from build123d import *

# Parameters (mm, degrees)
BOSS_EXTRU_1_DEPTH                    = 3.6
ESQUISSE2_W                           = 19.8
ESQUISSE2_H                           = 10.6
BOSS_EXTRU_2_DEPTH                    = 1.4
ESQUISSE3_W                           = 19.8
ESQUISSE3_H                           = 10.6
BOSS_EXTRU_3_DEPTH                    = 1.4
ESQUISSE4_W                           = 3.6
ESQUISSE4_H                           = 0.3
BOSS_EXTRU_4_DEPTH                    = 16.265607889
ESQUISSE5_W                           = 10.8
ESQUISSE5_H                           = 1.1
ENL_V_MAT_EXTRU_1_DEPTH               = 7.4
ESQUISSE6_W                           = 3.8
ESQUISSE6_H                           = 0.4
ENL_V_MAT_EXTRU_2_DEPTH               = 7.4
ESQUISSE7_W                           = 6.7
ESQUISSE7_H                           = 0.4
ENL_V_MAT_EXTRU_3_DEPTH               = 7.4
ESQUISSE8_W                           = 3.7
ESQUISSE8_H                           = 0.4
ENL_V_MAT_EXTRU_4_DEPTH               = 7.4
ENL_V_MAT_EXTRU_5_DEPTH               = 7.4
BOSS_EXTRU_5_DEPTH                    = 3.2
ESQUISSE11_W                          = 0.5
ESQUISSE11_H                          = 3.2
BOSS_EXTRU_6_DEPTH                    = 3.9
ESQUISSE12_W                          = 0.5
ESQUISSE12_H                          = 3.2
BOSS_EXTRU_7_DEPTH                    = 3.9
ESQUISSE13_W                          = 0.5
ESQUISSE13_H                          = 3.2
BOSS_EXTRU_8_DEPTH                    = 3.9
D_POUILLE1_ANGLE                      = 32.471192291
D_POUILLE2_ANGLE                      = 45
D_POUILLE3_ANGLE                      = 45
DIAM_TRE_DU_PER_AGE_2_35_2_35_1_D     = 2.35
DIAM_TRE_DU_PER_AGE_2_35_2_35_1_DEPTH = 6.4
CONG_1_R                              = 0.5
ESQUISSE16_R                          = 0.5
ENL_V_MAT_EXTRU_6_DEPTH               = 19.45


with BuildPart() as part:
    # Esquisse1 → Boss.-Extru.1 (new body)
    with BuildSketch(Plane(origin=(0, 0, -1.8), x_dir=(-1, 0, 0), z_dir=(0, 0, -1))):
        Polygon((7.1, 11.621125946), (6.88877818, 11.686563143), (6.8, 11.4), (6.8, 10.6), (-9.9, 10.6), (-9.9, 0), (9.9, 0), (9.9, 10.6), (7.1, 10.6), align=None)
    extrude(amount=-BOSS_EXTRU_1_DEPTH)

    # Esquisse2 → Boss.-Extru.2 (add)
    with BuildSketch(Plane(origin=(0, 0, -1.8), x_dir=(-1, 0, 0), z_dir=(0, 0, -1))):
        with Locations((0, 5.3)):
            Rectangle(ESQUISSE2_W, ESQUISSE2_H)
    extrude(amount=BOSS_EXTRU_2_DEPTH)

    # Esquisse3 → Boss.-Extru.3 (add)
    with BuildSketch(Plane.XY.offset(1.8)):
        with Locations((0, 5.3)):
            Rectangle(ESQUISSE3_W, ESQUISSE3_H)
    extrude(amount=BOSS_EXTRU_3_DEPTH)

    # Esquisse4 → Boss.-Extru.4 (add)
    with BuildSketch(Plane(origin=(-2.982033775, -0.923843615, 0), x_dir=(0, 0, -1), z_dir=(0.955210476, 0.295927265, 0))):
        with Locations((0, 13.051704831)):
            Rectangle(ESQUISSE4_W, ESQUISSE4_H)
    extrude(amount=BOSS_EXTRU_4_DEPTH)

    # Esquisse5 → Enlèv. mat.-Extru.1 (cut, through all)
    with BuildSketch(Plane.XY.offset(3.2)):
        with Locations((4.5, 10.05)):
            Rectangle(ESQUISSE5_W, ESQUISSE5_H)
    extrude(amount=-ENL_V_MAT_EXTRU_1_DEPTH, mode=Mode.SUBTRACT)

    # Esquisse6 → Enlèv. mat.-Extru.2 (cut, through all)
    with BuildSketch(Plane.XY.offset(3.2)):
        with Locations((8, 0.2)):
            Rectangle(ESQUISSE6_W, ESQUISSE6_H)
    extrude(amount=-ENL_V_MAT_EXTRU_2_DEPTH, mode=Mode.SUBTRACT)

    # Esquisse7 → Enlèv. mat.-Extru.3 (cut, through all)
    with BuildSketch(Plane.XY.offset(3.2)):
        with Locations((-0.05, 0.2)):
            Rectangle(ESQUISSE7_W, ESQUISSE7_H)
    extrude(amount=-ENL_V_MAT_EXTRU_3_DEPTH, mode=Mode.SUBTRACT)

    # Esquisse8 → Enlèv. mat.-Extru.4 (cut, through all)
    with BuildSketch(Plane.XY.offset(3.2)):
        with Locations((-8.05, 0.2)):
            Rectangle(ESQUISSE8_W, ESQUISSE8_H)
    extrude(amount=-ENL_V_MAT_EXTRU_4_DEPTH, mode=Mode.SUBTRACT)

    # Esquisse9 → Enlèv. mat.-Extru.5 (cut, through all)
    with BuildSketch(Plane.XY.offset(3.2)):
        with BuildLine():
            Line((-5.24, 1.73), (-4.36, 1.73))
            ThreePointArc((-4.36, 1.73), (-3.550086003, 2.914662921), (-4.387568187, 4.08))
            Line((-4.387568187, 4.08), (-5.212431813, 4.08))
            ThreePointArc((-5.212431813, 4.08), (-6.049913997, 2.914662921), (-5.24, 1.73))
        make_face()
    extrude(amount=-ENL_V_MAT_EXTRU_5_DEPTH, mode=Mode.SUBTRACT)

    # Esquisse10 → Boss.-Extru.5 (add)
    with BuildSketch(Plane(origin=(0, 0, -1.6), x_dir=(-1, 0, 0), z_dir=(0, 0, -1))):
        with BuildLine():
            Line((1.8, 10.6), (3.8, 10.6))
            Line((3.8, 10.6), (3.8, 11.263324958))
            ThreePointArc((3.8, 11.263324958), (2.8, 11.8), (1.8, 11.263324958))
            Line((1.8, 11.263324958), (1.8, 10.6))
        make_face()
    extrude(amount=-BOSS_EXTRU_5_DEPTH)

    # Esquisse11 → Boss.-Extru.6 (add)
    with BuildSketch(Plane.XZ.offset(-0.4)):
        with Locations((-8.3, 0)):
            Rectangle(ESQUISSE11_W, ESQUISSE11_H)
    extrude(amount=BOSS_EXTRU_6_DEPTH)

    # Esquisse12 → Boss.-Extru.7 (add)
    with BuildSketch(Plane.XZ.offset(-0.4)):
        with Locations((0.5, 0)):
            Rectangle(ESQUISSE12_W, ESQUISSE12_H)
    extrude(amount=BOSS_EXTRU_7_DEPTH)

    # Esquisse13 → Boss.-Extru.8 (add)
    with BuildSketch(Plane.XZ.offset(-0.4)):
        with Locations((7.8, 0)):
            Rectangle(ESQUISSE13_W, ESQUISSE13_H)
    extrude(amount=BOSS_EXTRU_8_DEPTH)

    # Dépouille1
    d_pouille1_faces = [part.faces().sort_by_distance(p)[0] for p in [
        (-0.9, 10.05, 0),
    ]]
    draft(d_pouille1_faces, Plane(origin=(-9.9, 10.6, 1.8), x_dir=(0, 0, 1), z_dir=(0, 1, 0)), D_POUILLE1_ANGLE)

    # Dépouille2
    d_pouille2_faces = [part.faces().sort_by_distance(p)[0] for p in [
        (6.1, 0.2, 0),
        (3.3, 0.2, 0),
    ]]
    draft(d_pouille2_faces, Plane(origin=(9.9, 0, 1.8), x_dir=(0, 0, -1), z_dir=(0, -1, 0)), D_POUILLE2_ANGLE)

    # Dépouille3
    d_pouille3_faces = [part.faces().sort_by_distance(p)[0] for p in [
        (-3.4, 0.2, 0),
        (-6.2, 0.2, 0),
    ]]
    draft(d_pouille3_faces, Plane(origin=(9.9, 0, 1.8), x_dir=(0, 0, -1), z_dir=(0, -1, 0)), D_POUILLE3_ANGLE)

    # Diamètre du perçage Ø2.35 (2.35)1
    with Locations(Plane.XY.offset(3.2)):
        with Locations((4.7, 2.9)):
            Hole(DIAM_TRE_DU_PER_AGE_2_35_2_35_1_D / 2, depth=DIAM_TRE_DU_PER_AGE_2_35_2_35_1_DEPTH)

    # Congé1
    cong_1_edges = [part.edges().sort_by_distance(p)[0] for p in [
        (-8.3, -3.5, -1.6),
        (-8.3, -3.5, 1.6),
        (0.5, -3.5, -1.6),
        (0.5, -3.5, 1.6),
        (7.8, -3.5, -1.6),
        (7.8, -3.5, 1.6),
    ]]
    fillet(cong_1_edges, radius=CONG_1_R)

    # Esquisse16 → Enlèv. mat.-Extru.6 (cut, through all)
    with BuildSketch(Plane.ZY.offset(8.55)):
        with Locations((0, -1.907139158)):
            Circle(ESQUISSE16_R)
    extrude(amount=-ENL_V_MAT_EXTRU_6_DEPTH, mode=Mode.SUBTRACT)


solid = part.part
Part model, mm, in its own coordinate system. A direction names the side the tool comes from. Coordinates: 2 decimals unless noted, no trailing zeros. Loops run counter-clockwise (first coordinate to the right, second up) from the corner with the lowest first, then second, coordinate; pieces in that order, holes last. Notation, with made-up numbers: M 40,18 L 84,18 A23 ccw 84,35 Z; hole C 76,74.5 d2. An arc over 180 degrees is marked long. Use a Markdown table: item, result. Add a question column.
Q1. Mould opens along Y. For faces 1 (the cylindrical face through (0.5, -2.35, 0.23)), 2 (the flat face through (0.75, -1, 0)) say: +Y half, -Y half, draft (parallel to the pull), parting line (faces both ways), or undercut.
Q2. Probe L1, parallel to X at y = -0.25, z = -1; L2, parallel to Y at x = 4.7, z = -1.25 (3 decimals); L3, parallel to X at y = 2.75, z = -0.5. List the from-to ranges inside material, lowest first.
Q3. Cut at A-A (y = -0.75). Write the cut outline in (x, z), and give its area (3 significant figures).
Q4. Pin check, flat tips, straight feed: P1, Ø1.9, axis at x = -6, z = 1.5, coming from the +Y side; P2, Ø1.4, axis at x = 5, z = 1, coming from the -Y side; P3, Ø1.6, axis at y = -2, z = 0, coming from the +X side. Stop position of each tip, or through.
Q5. Cut at C-C (x = 7.25). Write the cut outline in (y, z), and give its area (3 significant figures).
Q6. Cut at D-D (z = 0). Give the number of separate pieces and of enclosed holes in the cut face, and give its area (3 significant figures).
Q7. Cut at B-B (z = -2.25). Write the cut outline in (x, y) (3 decimals), and give its area (3 significant figures).
Q8. Which spindle directions (+Z, -Z, +X, -X, +Y, -Y) get a long thin tool onto all of the face, cutting with end or side? Do faces 3 (the flat face through (-0.545, 10.042, 0.045)), 4 (the flat face through (-6.8, 11, 0)), 5 (the flat face through (-7.1, 11, 0)). Say none if no direction does.
Worked out:
| question | item | result |
|---|---|---|
| 1 | face 1 | undercut |
| 1 | face 2 | draft |
| 2 | L1 | x = -8.55 to -8.05, 0.25 to 0.75, 7.55 to 8.05 |
| 2 | L2 | y = 0 to 1.725, 4.075 to 9.5, 14.963 to 15.277 |
| 2 | L3 | x = -9.9 to -6.04, -3.56 to 3.53, 5.87 to 9.9 |
| 3 | outline | M -8.55,-1.6 L -8.05,-1.6 L -8.05,1.6 L -8.55,1.6 Z; M 0.25,-1.6 L 0.75,-1.6 L 0.75,1.6 L 0.25,1.6 Z; M 7.55,-1.6 L 8.05,-1.6 L 8.05,1.6 L 7.55,1.6 Z |
| 3 | area | 4.80 mm2 |
| 4 | P1 | stops at y = 12.26 |
| 4 | P2 | stops at y = 0 |
| 4 | P3 | stops at x = 8.05 |
| 5 | outline | M 0.4,-3.2 L 9.5,-3.2 L 9.5,3.2 L 0.4,3.2 Z; M 15.75,-1.8 L 16.07,-1.8 L 16.07,1.8 L 15.75,1.8 Z |
| 5 | area | 59.4 mm2 |
| 6 | separate pieces | 4 |
| 6 | enclosed holes | 2 |
| 6 | area | 195 mm2 |
| 7 | outline | M -9.9,0.4 L -6.6,0.4 L -6.2,0 L -3.4,0 L -3,0.4 L 2.9,0.4 L 3.3,0 L 6.1,0 L 6.5,0.4 L 9.9,0.4 L 9.9,9.5 L -0.2,9.5 L -0.9,10.6 L -9.9,10.6 Z; hole M -5.24,1.73 L -4.36,1.73 A1.25 ccw -4.388,4.08 L -5.212,4.08 A1.25 ccw Z; hole C 4.7,2.9 d2.35 |
| 7 | area | 184 mm2 |
| 8 | face 3 | +Z, -Z, +X |
| 8 | face 4 | +Z, -Z |
| 8 | face 5 | +Z, -Z, -X, +Y |
